For this review, take the finished solid that the model builds, in its own axes (mm). Give positions to 0.01 mm unless a question says otherwise; leave off trailing zeros. Write each loop counter-clockwise with the first axis right and the second up, starting at its lowest first coordinate (ties: lowest second). Pieces come first, ordered by that corner, then holes. Notation, with made-up numbers: (49.5, 62) -> (61.5, 62) arc R31 ccw to (61.5, 96) -> close; hole circle Ø8 at (3, 18.5). An arc over 180 degrees is marked (long way). Return JSON: item names as keys, results as strings.
Autodesk Inventor part; units mm, degrees
ref_plane "YZ Plane" through (0, 0, 0) normal (1, 0, 0) x (0, 1, 0)
ref_plane "XZ Plane" through (0, 0, 0) normal (0, 1, 0) x (-1, 0, 0)
ref_plane "XY Plane" through (0, 0, 0) normal (0, 0, 1) x (1, 0, 0)
sketch "Boceto1" plane through (0, 0, 0) normal (0, 0, 1) x (1, 0, 0)
  circle A0 centre (100.65, -156.7) radius 1.65
  circle A1 centre (100.65, -148.3) radius 1.65
  circle A2 centre (100.65, 156.7) radius 1.65
  circle A3 centre (100.65, 148.3) radius 1.65
  line L0 (97.75, 145) -> (105.25, 145)
  line L1 (105.25, 145) -> (105.25, 160)
  line L2 (105.25, 160) -> (97.75, 160)
  line L3 (97.75, 160) -> (97.75, 180)
  line L4 (97.75, 180) -> (-109, 180)
  line L5 (-109, 160) -> (-115.3, 160)
  line L6 (-109, -160) -> (-109, -180)
  line L7 (-115.3, 146.9) -> (-109, 146.9)
  line L8 (-109, -146.9) -> (-115.3, -146.9)
  line L9 (-109, 180) -> (-109, 160)
  line L10 (-115.3, -160) -> (-109, -160)
  line L11 (-109, -180) -> (97.75, -180)
  line L12 (97.75, -180) -> (97.75, -160)
  line L13 (97.75, -160) -> (105.25, -160)
  line L14 (105.25, -160) -> (105.25, -145)
  line L15 (105.25, -145) -> (97.75, -145)
  line L16 (97.75, -145) -> (97.75, -142)
  line L17 (97.75, -142) -> (109, -142)
  line L18 (109, -142) -> (109, 142)
  line L19 (109, 142) -> (97.75, 142)
  line L20 (97.75, 142) -> (97.75, 145)
  line L21 (109, 180) -> (97.75, 180)
  line L22 (-109, -160) -> (-109, -180)
  line L23 (-109, -180) -> (-102.7, -180)
  line L24 (-109, -180) -> (109, -180)
  line L25 (109, -180) -> (109, 180)
  line L26 (109, 180) -> (-109, 180)
  line L27 (111, 142) -> (111, 180)
  line L28 (109, 182) -> (97.75, 182)
  line L29 (-109, -182) -> (-102.7, -182)
  line L30 (-111, -182) -> (111, -182)
  line L31 (111, -182) -> (111, 182)
  line L32 (111, 182) -> (-111, 182)
  circle A4 centre (-111.9, -156.3) radius 1.2
  circle A5 centre (-111.9, -150.6) radius 1.2
  circle A6 centre (-111.9, 156.3) radius 1.2
  circle A7 centre (-111.9, 150.6) radius 1.2
  line L33 (-115.3, 160) -> (-115.3, 146.9)
  line L34 (-109, 146.9) -> (-109, -146.9)
  line L35 (-115.3, -146.9) -> (-115.3, -160)
  line L36 (-109, 180) -> (-115.3, 180)
  line L37 (-109, -180) -> (-115.3, -180)
  line L38 (-115.3, 180) -> (109, 180)
  line L39 (109, 180) -> (109, -180)
  line L40 (109, -180) -> (-115.3, -180)
  line L41 (-115.3, -180) -> (-115.3, 180)
  line L42 (-117.3, 180) -> (-117.3, -182)
  line L43 (-117.3, -182) -> (109, -182)
  line L44 (-115.3, 182) -> (111, 182)
  line L45 (111, 182) -> (111, -180)
  line L46 (-117.3, 180) -> (-117.3, 182)
  line L47 (-117.3, 182) -> (-115.3, 182)
  point P0 (0, 0)
  dimension "d1" = 2
  dimension "d3" = 2
  dimension "d20" = 2
  dimension "d21" = 2
extrude "Extrusión1" add sketch "Boceto1" against normal blind 7.5 contours L0 L1 L2 L3 L21 L25 L19 L20 | L25 L24 L12 L13 L14 L15 L16 L17 | L9 L5 L41 L36 | L37 L41 L10 L6 | L7 L34 L8 L41 | L31 L30 L29 L43 L42 L46 L47 L44 L32 L28 L27
sketch "Boceto2" plane through (0, 0, 0) normal (0, 0, 1) x (1, 0, 0)
  line L0 (-117.3, -182) -> (111, -182)
  line L1 (111, -182) -> (111, 182)
  line L2 (111, 182) -> (-117.3, 182)
  line L3 (90.8, 170.8) -> (90.8, -176)
  line L4 (90.8, 170.8) -> (90.8, -176)
  line L5 (-19.4789, -176) -> (90.8, -176)
  line L6 (90.8, -176) -> (-99.7, -176)
  line L7 (-99.7, -176) -> (-99.7, 170.8)
  line L8 (-99.7, 170.8) -> (90.8, 170.8)
  line L9 (-117.3, 182) -> (-117.3, -182)
  line L10 (-105.5008, -176) -> (-99.7, -176)
  line L11 (-99.7, 170.8) -> (-105.5008, 170.8)
  line L12 (-109, 160) -> (-109, 180)
  line L13 (-109, 170.8) -> (-105, 170.8)
  line L14 (-105, 170.8) -> (-105, -176)
  point P0 (0, 0)
  dimension "d33" = 4
extrude "Extrusión2" add sketch "Boceto2" along normal blind 1.5
sketch "Boceto3" plane through (-111, -182, -7.5) normal (0, -1, 0) x (1, 0, 0)
  line L0 (222, 0) -> (-6.3, 0)
  line L1 (222, 0) -> (222, 9)
  line L2 (-6.3, 9) -> (222, 9)
  line L3 (-6.3, 0) -> (-6.3, 9)
  point P0 (111, 7.5)
extrude "Extrusión3" add sketch "Boceto3" along normal blind 5.2
sketch "Boceto5" plane through (0, 0, 1.5) normal (0, 0, 1) x (1, 0, 0)
  circle A0 centre (100.65, -156.7) radius 1.65
  circle A1 centre (100.65, -148.3) radius 1.65
  circle A2 centre (100.65, 156.7) radius 1.65
  circle A3 centre (100.65, 148.3) radius 1.65
  line L0 (97.75, 145) -> (105.25, 145)
  line L1 (105.25, 145) -> (105.25, 160)
  line L2 (105.25, 160) -> (97.75, 160)
  line L3 (97.75, 160) -> (97.75, 180)
  line L4 (97.75, 180) -> (-109, 180)
  line L5 (-109, 160) -> (-115.3, 160)
  line L6 (-109, -160) -> (-109, -180)
  line L7 (-115.3, 146.9) -> (-109, 146.9)
  line L8 (-109, -146.9) -> (-115.3, -146.9)
  line L9 (-109, 180) -> (-109, 160)
  line L10 (-115.3, -160) -> (-109, -160)
  line L11 (-109, -180) -> (97.75, -180)
  line L12 (97.75, -180) -> (97.75, -160)
  line L13 (97.75, -160) -> (105.25, -160)
  line L14 (105.25, -160) -> (105.25, -145)
  line L15 (105.25, -145) -> (97.75, -145)
  line L16 (97.75, -145) -> (97.75, -142)
  line L17 (97.75, -142) -> (109, -142)
  line L18 (109, -142) -> (109, 142)
  line L19 (109, 142) -> (97.75, 142)
  line L20 (97.75, 142) -> (97.75, 145)
  circle A4 centre (-111.9, -156.3) radius 1.2
  circle A5 centre (-111.9, -150.6) radius 1.2
  circle A6 centre (-111.9, 156.3) radius 1.2
  circle A7 centre (-111.9, 150.6) radius 1.2
  line L21 (-115.3, 160) -> (-115.3, 146.9)
  line L22 (-109, 146.9) -> (-109, -146.9)
  line L23 (-115.3, -146.9) -> (-115.3, -160)
  point P0 (0, 0)
hole "Agujero1" at (100.65, 148.3, 1.5) at (100.65, 156.7, 1.5) at (100.65, -156.7, 1.5) at (100.65, -148.3, 1.5) at (-111.9, -156.3, 1.5) at (-111.9, -150.6, 1.5) at (-111.9, 150.6, 1.5) at (-111.9, 156.3, 1.5) direction (0, 0, -1) diameter 2.4 end through all
sketch "Boceto6" plane through (0, 0, -7.5) normal (0, 0, -1) x (-1, 0, 0)
  line L0 (117.3, 182) -> (-111, 182)
  line L1 (-111, 182) -> (-111, -187.2)
  line L2 (117.3, -187.2) -> (-111, -187.2)
  line L3 (117.3, 182) -> (117.3, -187.2)
  line L4 (-97.75, 160) -> (-97.75, 180)
  line L5 (-97.75, 180) -> (109, 180)
  line L6 (109, 180) -> (109, 160)
  line L7 (109, 160) -> (115.3, 160)
  line L8 (115.3, 160) -> (115.3, 146.9)
  line L9 (115.3, 146.9) -> (109, 146.9)
  line L10 (109, 146.9) -> (109, -146.9)
  line L11 (109, -146.9) -> (115.3, -146.9)
  line L12 (115.3, -146.9) -> (115.3, -160)
  line L13 (115.3, -160) -> (109, -160)
  line L14 (109, -160) -> (109, -180)
  line L15 (109, -180) -> (-97.75, -180)
  line L16 (-97.75, -180) -> (-97.75, -160)
  line L17 (-97.75, -160) -> (-105.25, -160)
  line L18 (-105.25, -160) -> (-105.25, -145)
  line L19 (-105.25, -145) -> (-97.75, -145)
  line L20 (-97.75, -145) -> (-97.75, -142)
  line L21 (-97.75, -142) -> (-109, -142)
  line L22 (-109, -142) -> (-109, 142)
  line L23 (-109, 142) -> (-97.75, 142)
  line L24 (-97.75, 142) -> (-97.75, 145)
  line L25 (-97.75, 145) -> (-105.25, 145)
  line L26 (-105.25, 145) -> (-105.25, 160)
  line L27 (-105.25, 160) -> (-97.75, 160)
  line L28 (117.3, 182) -> (117.3, -187.2)
  line L29 (117.3, 182) -> (-111, 182)
  line L30 (-111, 182) -> (-111, -187.2)
  line L31 (117.3, -187.2) -> (-111, -187.2)
  line L32 (109.5, 160.5) -> (109.5, 180.5)
  line L33 (109.5, 180.5) -> (-98.25, 180.5)
  line L34 (-98.25, 180.5) -> (-98.25, 160.5)
  line L35 (-98.25, 160.5) -> (-105.75, 160.5)
  line L36 (-105.75, 160.5) -> (-105.75, 144.5)
  line L37 (-105.75, 144.5) -> (-98.25, 144.5)
  line L38 (-98.25, 144.5) -> (-98.25, 142.5)
  line L39 (-98.25, 142.5) -> (-109.5, 142.5)
  line L40 (-109.5, 142.5) -> (-109.5, -142.5)
  line L41 (-109.5, -142.5) -> (-98.25, -142.5)
  line L42 (-98.25, -142.5) -> (-98.25, -144.5)
  line L43 (-98.25, -144.5) -> (-105.75, -144.5)
  line L44 (-105.75, -144.5) -> (-105.75, -160.5)
  line L45 (-105.75, -160.5) -> (-98.25, -160.5)
  line L46 (-98.25, -160.5) -> (-98.25, -180.5)
  line L47 (-98.25, -180.5) -> (109.5, -180.5)
  line L48 (109.5, -180.5) -> (109.5, -160.5)
  line L49 (109.5, -160.5) -> (115.8, -160.5)
  line L50 (115.8, -160.5) -> (115.8, -146.4)
  line L51 (115.8, -146.4) -> (109.5, -146.4)
  line L52 (109.5, -146.4) -> (109.5, 146.4)
  line L53 (109.5, 146.4) -> (115.8, 146.4)
  line L54 (115.8, 146.4) -> (115.8, 160.5)
  line L55 (115.8, 160.5) -> (109.5, 160.5)
  dimension "d22" = 0.5
extrude "Extrusión4" cut sketch "Boceto6" against normal blind 7.5 contours L55 L54 L53 L52 L51 L50 L49 L48 L47 L46 L45 L44 L43 L42 L41 L40 L39 L38 L37 L36 L35 L34 L33 L32
fillet "Empalme1" radius 2 5 edges at (-117.3, 182, 0.75) (-117.3, 182, -3.75) (111, 182, -3) (111, -187.2, -3) (-117.3, -187.2, -3)
sketch "Boceto7" plane through (0, 0, -7.5) normal (0, 0, -1) x (-1, 0, 0)
  arc A0 (117.3, 7) -> (114.3, 10) centre (114.3, 7) ccw
  line L0 (114.3, 10) -> (100.3, 10)
  arc A1 (100.3, 10) -> (97.3, 7) centre (100.3, 7) ccw
  line L1 (97.3, 7) -> (97.3, -7)
  arc A2 (97.3, -7) -> (100.3, -10) centre (100.3, -7) ccw
  line L2 (100.3, -10) -> (114.3, -10)
  arc A3 (114.3, -10) -> (117.3, -7) centre (114.3, -7) ccw
  line L3 (117.3, -7) -> (117.3, 7)
  circle A4 centre (103.3, -5) radius 1
  circle A5 centre (113.3, 5) radius 1
  circle A6 centre (103.3, 5) radius 1
  circle A7 centre (113.3, -5) radius 1
  circle A8 centre (113.3, 5) radius 1
  point P0 (0, 0)
hole "Agujero2" at (-113.3, 5, -7.5) at (-113.3, -5, -7.5) direction (0, 0, 1) diameter 3 depth 6
split "Dividir4" plane through (0, 0, 0) removes the side toward (0, -1, 0)
sketch "Boceto8" plane through (111, 180, 1.5) normal (1, 0, 0) x (0, 0, -1)
  circle A0 centre (5.1, -175) radius 1.2
  point P0 (1.5, -180)
hole "Agujero3" at (111, 5, -3.6) direction (-1, 0, 0) diameter 2.4 depth 8 tip angle 118
properties part number "MarcoDerecho"
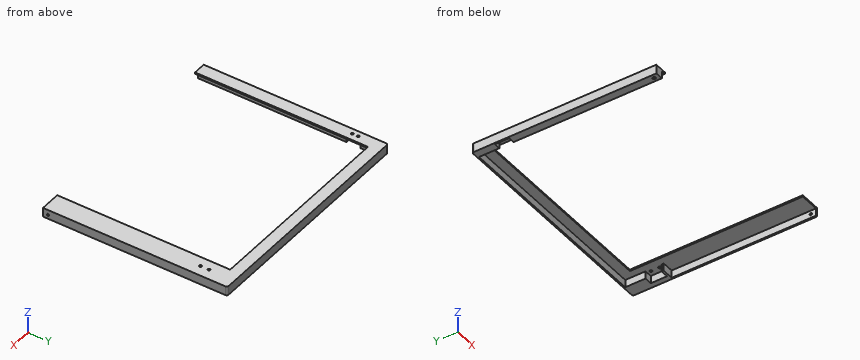
1. To check wall thickness, follow probe 1 along Y at (x, z) = (100.65, 0.35); probe 2 along Y at (x, z) = (-113.3, -3.85); probe 3 along X at (y, z) = (148.3, 0.95). State the ranges of each line that lie inside material, in increasing order.
Results found:
{"probe 1": "y = 0 to 147.1, 149.5 to 155.5, 157.9 to 182", "probe 2": "y = 0 to 3.5, 6.5 to 146.4, 160.5 to 182", "probe 3": "x = -117.3 to -105, 90.8 to 99.45, 101.85 to 111"}
2. Add section B-B, the plane x = 11.5. State the section outline as (y, z) points.
Results found:
{"outline": "(170.8, 0) -> (180.5, 0) -> (180.5, -7.5) -> (182, -7.5) -> (182, 1.5) -> (170.8, 1.5) -> close"}
3. For pin 1 (3 mm diameter, centred on x = 100.65, y = 156.7, fed in from +Z); pin 2 (1.6 mm diameter, centred on x = -49.5, z = 1, fed in from -Y); pin 3 (2 mm diameter, centred on x = -111.9, y = 156.3, fed in from +Z), all flat-tipped, find the tip position at first contact; note any pin that passes through.
Results found:
{"pin 1": "stops at z = 1.5", "pin 2": "stops at y = 170.8", "pin 3": "passes through"}
4. Add section A-A, the plane y = 128.5. State the section outline as (x, z) points, plus the area to 4 significant figures.
Results found:
{"outline": "(-117.3, -7.5) -> (-109.5, -7.5) -> (-109.5, 0) -> (-105, 0) -> (-105, 1.5) -> (-117.3, 1.5) -> close; (90.8, 0) -> (109.5, 0) -> (109.5, -7.5) -> (111, -7.5) -> (111, 1.5) -> (90.8, 1.5) -> close", "area": "118.5 mm²"}
